Here's how the part is built. I have some questions about the finished solid (model axes, mm). A direction names the side the tool comes from. Round coordinates to 2 decimals unless told otherwise and drop trailing zeros. Loops run counter-clockwise (first coordinate to the right, second up) from the corner with the lowest first, then second, coordinate; pieces in that order, holes last. Notation, with made-up numbers: M 38,-10 L 59,-10 A22 ccw 59,24 Z; hole C 18,65.25 d11. An arc over 180 degrees is marked long. Answer as a JSON object with one key per item and string values.
from build123d import *

# Parameters (mm, degrees)
SKETCH1_R                = 11.1125
BOSS_EXTRUDE1_DEPTH      = 38.1
BOSS_EXTRUDE2_DEPTH      = 12.7
BOSS_EXTRUDE2_DEPTH_BACK = 12.7
SKETCH2_W                = 9.525
SKETCH2_H                = 31.75
BOSS_EXTRUDE3_DEPTH      = 12.7
BOSS_EXTRUDE3_DEPTH_BACK = 12.7
SKETCH3_W                = 63.5
SKETCH3_H                = 12.7
BOSS_EXTRUDE4_DEPTH      = 12.7
BOSS_EXTRUDE4_DEPTH_BACK = 12.7
SKETCH4_W                = 9.525
SKETCH4_H                = 60.2996
BOSS_EXTRUDE5_DEPTH      = 12.7
BOSS_EXTRUDE5_DEPTH_BACK = 12.7
SKETCH5_W                = 25.4
SKETCH5_H                = 9.525


with BuildPart() as part:
    # Sketch1 → Boss-Extrude1 (new body)
    with BuildSketch(Plane(origin=(0, 0, 0), x_dir=(0, 0, -1), z_dir=(1, 0, 0))):
        Circle(SKETCH1_R)
    extrude(amount=-BOSS_EXTRUDE1_DEPTH)

    # Sketch2 → Boss-Extrude2 (add, two sides: drawn at the far end of the back side and taken through both)
    with BuildSketch(Plane.XY.offset(-BOSS_EXTRUDE2_DEPTH_BACK)):
        with Locations((4.7625, 4.7625)):
            Rectangle(SKETCH2_W, SKETCH2_H)
    extrude(amount=BOSS_EXTRUDE2_DEPTH + BOSS_EXTRUDE2_DEPTH_BACK)

    # Sketch3 → Boss-Extrude3 (add, two sides: drawn at the far end of the back side and taken through both)
    with BuildSketch(Plane.XY.offset(-BOSS_EXTRUDE3_DEPTH_BACK)):
        with Locations((-22.225, 26.9875)):
            Rectangle(SKETCH3_W, SKETCH3_H)
    extrude(amount=BOSS_EXTRUDE3_DEPTH + BOSS_EXTRUDE3_DEPTH_BACK)

    # Sketch4 → Boss-Extrude4 (add, two sides: drawn at the far end of the back side and taken through both)
    with BuildSketch(Plane.XY.offset(-BOSS_EXTRUDE4_DEPTH_BACK)):
        with Locations((-49.2125, 50.7873)):
            Rectangle(SKETCH4_W, SKETCH4_H)
    extrude(amount=BOSS_EXTRUDE4_DEPTH + BOSS_EXTRUDE4_DEPTH_BACK)

    # Sketch5 → Boss-Extrude5 (add, two sides: drawn at the far end of the back side and taken through both)
    with BuildSketch(Plane.XY.offset(-BOSS_EXTRUDE5_DEPTH_BACK)):
        with Locations((-41.275, 76.1746)):
            Rectangle(SKETCH5_W, SKETCH5_H)
    extrude(amount=BOSS_EXTRUDE5_DEPTH + BOSS_EXTRUDE5_DEPTH_BACK)


solid = part.part
Item 1: For faces 5 (the face through (0, 12, 0)), 6 (the face through (-38.1, 0, 0)), 7 (the face through (-28.575, 76, 0)), 8 (the face through (-27, 20.638, 0)), which set-ups out of +Z, -Z, +X, -X, +Y, -Y let a thin tool reach every point of the face, with its end or its side?
Solution:
{"face 5": "-X", "face 6": "+Z, -Z, -X, -Y", "face 7": "+Z, -Z, +X, +Y", "face 8": "+Z, -Z, -X"}
Item 2: I want a section at A-A on x = -33. List the corners of the cut face in (y, z) for me (1 decimal).
Solution:
{"outline": "C 0,0 d22.2; M 20.6,-12.7 L 33.3,-12.7 L 33.3,12.7 L 20.6,12.7 Z; M 71.4,-12.7 L 80.9,-12.7 L 80.9,12.7 L 71.4,12.7 Z"}
Item 3: For P1, Ø5, axis at y = 38, z = -7.5, coming from the +X side; P2, Ø12.5, axis at y = 5.5, z = 0, coming from the -X side; P3, Ø5, axis at y = 76, z = -0.5, coming from the +X side (3 decimals), each with a flat end and sliding along its axis, tell me the tip position at first contact or that it passes through.
Solution:
{"P1": "stops at x = -44.45", "P2": "stops at x = -38.1", "P3": "stops at x = -28.575"}
Item 4: I want a section at D-D on x = 6. List the corners of the cut face in (y, z) for me, plus the area to 3 significant figures.
Solution:
{"outline": "M -11.11,-12.7 L 33.34,-12.7 L 33.34,12.7 L -11.11,12.7 Z", "area": "1,130 mm2"}
Item 5: I want a section at B-B on y = 0. List the corners of the cut face in (x, z) for me (1 decimal), plus the area to 3 significant figures.
Solution:
{"outline": "M -38.1,-11.1 L 0,-11.1 L 0,-12.7 L 9.5,-12.7 L 9.5,12.7 L 0,12.7 L 0,11.1 L -38.1,11.1 Z", "area": "1,090 mm2"}
Item 6: We'd pull the mould along Y, two halves only. Please class faces 1 (the face through (-41, 80.937, 0)), 2 (the face through (-44.45, 52, 0)), 3 (the face through (9.525, 11, 0)), 4 (the face through (-37, 71.412, 0)): +Y half, -Y half, draft (parallel to the pull), parting line (faces both ways), or undercut.
Solution:
{"face 1": "+Y half", "face 2": "undercut", "face 3": "draft", "face 4": "undercut"}
Item 7: If I drill on L1, parallel to Y at x = -13, z = -0.5; L2, parallel to Y at x = -42, z = -2.25; L3, parallel to X at y = 76.5, z = -10.25 (3 decimals), over which ranges is the centre line in solid material (lowest first)? Write a range as from..to.
Solution:
{"L1": "y = -11.1..11.1, 20.64..33.34", "L2": "y = 20.64..33.34, 71.41..80.94", "L3": "x = -53.975..-28.575"}
